from build123d import *

# Parameters (mm, degrees)
SKETCH1_W               = 120
SKETCH1_H               = 38
SKETCH1_W_2             = 41
SKETCH1_H_2             = 20
BOSS_EXTRUDE1_DEPTH     = 11
FILLET1_RADIUS          = 19
FILLET1_LENGTH          = 11
BOSS_EXTRUDE2_START     = 8
BOSS_EXTRUDE2_DEPTH     = 8
FILLET2_R               = 16
CUT_EXTRUDE2_DEPTH      = 66.741919656
CUT_EXTRUDE2_DEPTH_BACK = 66.741919656
BOSS_EXTRUDE3_START     = 8
BOSS_EXTRUDE3_OUTLINE_W = 32
BOSS_EXTRUDE3_OUTLINE_H = 8
BOSS_EXTRUDE3_DEPTH     = 49
SKETCH8_W               = 52
SKETCH8_H               = 38
BOSS_EXTRUDE4_DEPTH     = 8
SKETCH9_W               = 27
SKETCH9_H               = 38
CUT_EXTRUDE3_DEPTH      = 5
BOSS_EXTRUDE5_START     = -2
SKETCH11_W              = 41
SKETCH11_H              = 20
BOSS_EXTRUDE5_DEPTH     = 2
SKETCH13_R              = 6.5
CUT_EXTRUDE6_DEPTH      = 8
FILLET7_R               = 6
SKETCH25_R              = 2.15
CUT_EXTRUDE13_DEPTH     = 66.741919805
SKETCH10_W              = 38.2
SKETCH10_H              = 20
CUT_EXTRUDE14_DEPTH     = 74.518705262
BOSS_EXTRUDE6_DEPTH     = 1.5
LPATTERN1_COUNT         = 2
LPATTERN1_PITCH         = 39.5
SKETCH27_W              = 10
SKETCH27_H              = 8
BOSS_EXTRUDE7_DEPTH     = 27
FILLET8_R               = 3
CUT_EXTRUDE15_REACH     = 114.349
SKETCH28_R              = 2.15


# Read off the part's stored shape, not the designer's step: Boss-Extrude3
# Some blends are built 0.0001 mm under size
with BuildPart() as part:
    # Sketch1 → Boss-Extrude1 (new body)
    with BuildSketch(Plane.XY):
        Rectangle(SKETCH1_W, SKETCH1_H)
        with Locations((-24.5, 0)):
            Rectangle(SKETCH1_W_2, SKETCH1_H_2, mode=Mode.SUBTRACT)
    extrude(amount=BOSS_EXTRUDE1_DEPTH)

    # Fillet1: full round fillet: the end face becomes a half cylinder, R = half its width
    fillet1_face = Plane((-60, 0, 5.5), x_dir=(0, 0, 1), z_dir=(-1, 0, 0))  # on the end face: x along it, z out of the body
    fillet1_slab = fillet1_face.offset(-FILLET1_RADIUS / 2) * Box(FILLET1_LENGTH, 2 * FILLET1_RADIUS, FILLET1_RADIUS, mode=Mode.PRIVATE)  # the body's end, R deep
    fillet1_round = Plane((-41, 0, 5.5), x_dir=(-1, 0, 0), z_dir=(0, 0, 1)) * Cylinder(FILLET1_RADIUS, FILLET1_LENGTH, mode=Mode.PRIVATE)  # its axis R under the face
    add(fillet1_slab - fillet1_round, mode=Mode.SUBTRACT)

    # Sketch5 → Boss-Extrude2 (add)
    with BuildSketch(Plane.XY.offset(11).offset(BOSS_EXTRUDE2_START)):
        with BuildLine():
            Line((60, 19), (-41, 19))
            ThreePointArc((-41, 19), (-60, 0), (-41, -19))
            Line((-41, -19), (60, -19))
            Line((60, -19), (60, 19))
        make_face()
        with BuildLine():
            Line((57, 16), (-41, 16))
            ThreePointArc((-41, 16), (-57, 0), (-41, -16))
            Line((-41, -16), (57, -16))
            Line((57, -16), (57, 16))
        make_face(mode=Mode.SUBTRACT)
    extrude(amount=-BOSS_EXTRUDE2_DEPTH)

    # Fillet2
    fillet2_edges = [part.edges().sort_by_distance(p)[0] for p in [
        (57, 16, 15),
        (57, -16, 15),
    ]]
    fillet(fillet2_edges, radius=FILLET2_R - 0.0001)  # a hair under: the kernel refuses the full size

    # Sketch6 → Cut-Extrude2 (cut, two sides: drawn at the far end of the back side and taken through both)
    with BuildSketch(Plane(origin=(0, 0, 0), x_dir=(1, 0, 0), z_dir=(0, 1, 0)).offset(-CUT_EXTRUDE2_DEPTH_BACK)):
        with BuildLine():
            add(Edge.make_bspline(
                [(-60, -13.666666667), (-50.023022061, -12.774335398), (-44.35489615, -13.481329797), (-34.284055631, -17.771751053), (-23.960245459, -19), (-20, -19)],
                knots=[0, 0, 0, 0, 0.415410377, 0.639728072, 1, 1, 1, 1], degree=3))
            Line((-20, -19), (-60, -19))
            Line((-60, -19), (-60, -13.666666667))
        make_face()
    extrude(amount=CUT_EXTRUDE2_DEPTH + CUT_EXTRUDE2_DEPTH_BACK, mode=Mode.SUBTRACT)

    # Boss-Extrude3 outline → Boss-Extrude3 (add)
    with BuildSketch(Plane.YZ.offset(BOSS_EXTRUDE3_START)):
        with Locations((0, 15)):
            Rectangle(BOSS_EXTRUDE3_OUTLINE_W, BOSS_EXTRUDE3_OUTLINE_H)
    extrude(amount=BOSS_EXTRUDE3_DEPTH)

    # Sketch8 → Boss-Extrude4 (add)
    with BuildSketch(Plane(origin=(0, 0, 0), x_dir=(-1, 0, 0), z_dir=(0, 0, -1))):
        with Locations((-34, 0)):
            Rectangle(SKETCH8_W, SKETCH8_H)
    extrude(amount=BOSS_EXTRUDE4_DEPTH)

    # Sketch9 → Cut-Extrude3 (cut)
    with BuildSketch(Plane(origin=(60, 0, 0), x_dir=(0, 0, -1), z_dir=(1, 0, 0))):
        with Locations((-5.5, 0)):
            Rectangle(SKETCH9_W, SKETCH9_H)
    extrude(amount=-CUT_EXTRUDE3_DEPTH, mode=Mode.SUBTRACT)

    # Sketch11 → Boss-Extrude5 (add)
    with BuildSketch(Plane(origin=(0, 0, 0), x_dir=(-1, 0, 0), z_dir=(0, 0, -1)).offset(BOSS_EXTRUDE5_START)):
        with BuildLine():
            Line((-8, 19), (-8, -19))
            Line((-8, -19), (41, -19))
            ThreePointArc((41, -19), (60, 0), (41, 19))
            Line((41, 19), (-8, 19))
        make_face()
        with Locations((24.5, 0)):
            Rectangle(SKETCH11_W, SKETCH11_H, mode=Mode.SUBTRACT)
    extrude(amount=BOSS_EXTRUDE5_DEPTH)

    # Sketch13 → Cut-Extrude6 (cut)
    with BuildSketch(Plane(origin=(55, 0, 0), x_dir=(0, 0, -1), z_dir=(1, 0, 0))):
        with Locations(Location((-5.5, 5.3, 0), (0, 0, 90))):
            Circle(SKETCH13_R)
    extrude(amount=-CUT_EXTRUDE6_DEPTH, mode=Mode.SUBTRACT)

    # Fillet7
    fillet7_edges = [part.edges().sort_by_distance(p)[0] for p in [
        (8, 0, 0),
    ]]
    fillet(fillet7_edges, radius=FILLET7_R)

    # Sketch25 → Cut-Extrude13 (cut, through all)
    with BuildSketch(Plane.XY.offset(11)):
        with Locations((-49.85, 5)):
            Circle(SKETCH25_R)
        with Locations((-49.85, -5)):
            Circle(SKETCH25_R)
        with Locations((0.05, -5)):
            Circle(SKETCH25_R)
        with Locations((0.05, 5)):
            Circle(SKETCH25_R)
    extrude(amount=-CUT_EXTRUDE13_DEPTH, mode=Mode.SUBTRACT)

    # Sketch10 → Cut-Extrude14 (cut, through all)
    with BuildSketch(Plane.XZ.offset(19)):
        with Locations((35.9, 5.5)):
            Rectangle(SKETCH10_W, SKETCH10_H)
    extrude(amount=-CUT_EXTRUDE14_DEPTH, mode=Mode.SUBTRACT)

    # Sketch26 → Boss-Extrude6 (add)
    with BuildSketch(Plane.XZ.offset(19)):
        Polygon((8, -8), (55, -8), (55, -4.5), (16.8, -4.5), (16.8, 15.5), (55, 15.5), (55, 19), (8, 19), (8, -6), align=None)
    boss_extrude6 = extrude(amount=BOSS_EXTRUDE6_DEPTH)

    # LPattern1: Boss-Extrude6 ×2
    with Locations(*[(0, i * LPATTERN1_PITCH, 0) for i in range(1, LPATTERN1_COUNT)]):
        add(boss_extrude6)

    # Sketch27 → Boss-Extrude7 (add, through all)
    with BuildSketch(Plane.XY.offset(19)):
        with Locations((42, 24.5)):
            Rectangle(SKETCH27_W, SKETCH27_H)
        with Locations((42, -24.5)):
            Rectangle(SKETCH27_W, SKETCH27_H)
    extrude(amount=-BOSS_EXTRUDE7_DEPTH)

    # Fillet8
    # the kernel refuses this fillet: 3 mm, written as the material it takes off along each edge
    with BuildSketch(Plane(origin=(55, -28, 19), x_dir=(-1, 0, 0), z_dir=(0, 1, 0)), Plane(origin=(55, 28, -8), x_dir=(-1, 0, 0), z_dir=(0, -1, 0)), Plane(origin=(55, -28, 15.5), x_dir=(0, 0, 1), z_dir=(0, 1, 0))) as fillet8_piece_1:
        with BuildLine():
            CenterArc((FILLET8_R, -FILLET8_R), FILLET8_R, 90, 90)
            Line((0, -FILLET8_R), (0, 0))
            Line((0, 0), (FILLET8_R, 0))
        make_face()
    extrude(amount=56, mode=Mode.SUBTRACT)
    with BuildSketch(Plane(origin=(55, 28, -4.5), x_dir=(-1, 0, 0), z_dir=(0, -1, 0))) as fillet8_piece_2:
        with BuildLine():
            CenterArc((FILLET8_R, FILLET8_R), FILLET8_R, 180, 90)
            Line((0, FILLET8_R), (0, 0))
            Line((0, 0), (FILLET8_R, 0))
        make_face()
    extrude(amount=56, mode=Mode.SUBTRACT)
    with BuildSketch(Plane(origin=(47, 36, -8), x_dir=(-1, 0, 0), z_dir=(0, -1, 0)), Plane(origin=(47, -36, 19), x_dir=(-1, 0, 0), z_dir=(0, 1, 0))) as fillet8_piece_3:
        with BuildLine():
            CenterArc((FILLET8_R, -FILLET8_R), FILLET8_R, 90, 90)
            Line((0, -FILLET8_R), (0, 0))
            Line((0, 0), (FILLET8_R, 0))
        make_face()
    extrude(amount=15.5, mode=Mode.SUBTRACT)
    with BuildSketch(Plane(origin=(29.5, 28.5, -8), x_dir=(0, -1, 0), z_dir=(1, 0, 0)), Plane(origin=(29.5, -28.5, 19), x_dir=(0, 1, 0), z_dir=(1, 0, 0))) as fillet8_piece_4:
        with BuildLine():
            CenterArc((FILLET8_R, -FILLET8_R), FILLET8_R, 90, 90)
            Line((0, -FILLET8_R), (0, 0))
            Line((0, 0), (FILLET8_R, 0))
        make_face()
    extrude(amount=25, mode=Mode.SUBTRACT)
    with BuildSketch(Plane(origin=(47, 36, 19), x_dir=(-1, 0, 0), z_dir=(0, -1, 0)), Plane(origin=(47, -36, -8), x_dir=(-1, 0, 0), z_dir=(0, 1, 0))) as fillet8_piece_5:
        with BuildLine():
            CenterArc((FILLET8_R, FILLET8_R), FILLET8_R, 180, 90)
            Line((0, FILLET8_R), (0, 0))
            Line((0, 0), (FILLET8_R, 0))
        make_face()
    extrude(amount=15.5, mode=Mode.SUBTRACT)
    with BuildSketch(Plane(origin=(29.5, 28.5, 19), x_dir=(0, -1, 0), z_dir=(1, 0, 0)), Plane(origin=(29.5, -28.5, -8), x_dir=(0, 1, 0), z_dir=(1, 0, 0))) as fillet8_piece_6:
        with BuildLine():
            CenterArc((FILLET8_R, FILLET8_R), FILLET8_R, 180, 90)
            Line((0, FILLET8_R), (0, 0))
            Line((0, 0), (FILLET8_R, 0))
        make_face()
    extrude(amount=25, mode=Mode.SUBTRACT)

    # Sketch28 → Cut-Extrude15 (cut, up to next)
    with BuildSketch(Plane(origin=(47, 0, 0), x_dir=(0, 0, -1), z_dir=(1, 0, 0)), mode=Mode.PRIVATE) as cut_extrude15_sk1:
        with Locations((-10.5, 25.35)):
            Circle(SKETCH28_R)
    cut_extrude15_tool1 = extrude(cut_extrude15_sk1.sketch, amount=-CUT_EXTRUDE15_REACH, mode=Mode.PRIVATE) & part.part
    # Sketch28 → Cut-Extrude15 (cut, up to next)
    with BuildSketch(Plane(origin=(47, 0, 0), x_dir=(0, 0, -1), z_dir=(1, 0, 0)), mode=Mode.PRIVATE) as cut_extrude15_sk2:
        with Locations((-0.5, 25.35)):
            Circle(SKETCH28_R)
    cut_extrude15_tool2 = extrude(cut_extrude15_sk2.sketch, amount=-CUT_EXTRUDE15_REACH, mode=Mode.PRIVATE) & part.part
    # Sketch28 → Cut-Extrude15 (cut, up to next)
    with BuildSketch(Plane(origin=(47, 0, 0), x_dir=(0, 0, -1), z_dir=(1, 0, 0)), mode=Mode.PRIVATE) as cut_extrude15_sk3:
        with Locations((-0.5, -25.35)):
            Circle(SKETCH28_R)
    cut_extrude15_tool3 = extrude(cut_extrude15_sk3.sketch, amount=-CUT_EXTRUDE15_REACH, mode=Mode.PRIVATE) & part.part
    # Sketch28 → Cut-Extrude15 (cut, up to next)
    with BuildSketch(Plane(origin=(47, 0, 0), x_dir=(0, 0, -1), z_dir=(1, 0, 0)), mode=Mode.PRIVATE) as cut_extrude15_sk4:
        with Locations((-10.5, -25.35)):
            Circle(SKETCH28_R)
    cut_extrude15_tool4 = extrude(cut_extrude15_sk4.sketch, amount=-CUT_EXTRUDE15_REACH, mode=Mode.PRIVATE) & part.part
    add(cut_extrude15_tool1.solids().sort_by_distance((47, 25.35, 10.5))[0], mode=Mode.SUBTRACT)
    add(cut_extrude15_tool2.solids().sort_by_distance((47, 25.35, 0.5))[0], mode=Mode.SUBTRACT)
    add(cut_extrude15_tool3.solids().sort_by_distance((47, -25.35, 0.5))[0], mode=Mode.SUBTRACT)
    add(cut_extrude15_tool4.solids().sort_by_distance((47, -25.35, 10.5))[0], mode=Mode.SUBTRACT)


solid = part.part
Geometry: final body of the model. Coordinates: model frame, mm. A direction names the side the tool comes from. Coordinates: 2 decimals unless noted, no trailing zeros. Order: outer loops, then holes, each group sorted by start corner. A loop starts at its lowest first (then second) coordinate and runs counter-clockwise, first axis right, second up.
1) Set-up query: faces 4 (the cylindrical face through (46.14, 23.67, 18.1)), 5 (the cylindrical face through (53.64, -0.29, 15.99)), 6 (the flat face through (-45, 0, 5)), 7 (the cylindrical face through (46.14, -23.67, -7.1)). Return all of +Z, -Z, +X, -X, +Y, -Y with unobstructed straight access to the full face (end or side cutting, diameter ignored); none if empty.
Result sheet:
face 4: +Z, +X, +Y
face 5: +X, +Y, -Y
face 6: +Z, -Z
face 7: -Z, +X, -Y
2) Section C-C (x = 33.5). Return loops of the section in (y, z), then the cut area to 3 significant figures.
Result sheet:
outline: (-20.5, -8) - (20.5, -8) - (20.5, -4.5) - (-20.5, -4.5) - close; (-20.5, 15.5) - (20.5, 15.5) - (20.5, 19) - (-20.5, 19) - close
area: 287 mm2
3) Ray query, probe 1 along Y at (x, z) = (0.05, 7.25); probe 2 along Z at (x, y) = (27.5, -11); probe 3 along Y at (x, z) = (-49.85, 5). Return the intervals inside material, ascending.
Result sheet:
probe 1: y = -19 to -7.15, -2.85 to 2.85, 7.15 to 19
probe 2: z = -8 to -4.5, 15.5 to 19
probe 3: y = -16.81 to -7.15, -2.85 to 2.85, 7.15 to 16.81
4) Section A-A (z = 5). Return loops of the section in (x, y).
Result sheet:
outline: (-41, -19) - (8, -19) - (8, -20.5) - (16.8, -20.5) - (16.8, 20.5) - (8, 20.5) - (8, 19) - (-41, 19) arc R19 ccw to start; (37, -28.5) - (47, -28.5) - (47, -20.5) - (37, -20.5) - close; (37, 20.5) - (47, 20.5) - (47, 28.5) - (37, 28.5) - close; hole circle Ø4.3 at (-49.85, -5); hole circle Ø4.3 at (-49.85, 5); hole (-45, -10) - (-4, -10) - (-4, 10) - (-45, 10) - close; hole circle Ø4.3 at (0.05, -5); hole circle Ø4.3 at (0.05, 5)
5) Section B-B (x = 0.05). Return loops of the section in (y, z).
Result sheet:
outline: (-19, 0) - (-7.15, 0) - (-7.15, 11) - (-16, 11) - (-16, 19) - (-19, 19) - close; (-2.85, 0) - (2.85, 0) - (2.85, 11) - (-2.85, 11) - close; (7.15, 0) - (19, 0) - (19, 19) - (16, 19) - (16, 11) - (7.15, 11) - close
6) Draft query along Y for faces 1 (the cylindrical face through (53.6, 0.29, -7.54)), 2 (the flat face through (16, 20.5, 6)), 3 (the flat face through (35, 0, -4.5)). Return one class per face: released by +Y, released by -Y, zero draft, split by the parting line, or undercut.
Result sheet:
face 1: zero draft
face 2: released by +Y
face 3: undercut
7) First-contact query: P1, Ø6, axis at x = -14.5, y = 16.5, coming from the -Z side; P2, Ø3.5, axis at x = 0.05, y = 5, coming from the +Z side; P3, Ø1, axis at x = 12, z = 1, coming from the -Y side; P4, Ø7, axis at x = 0.05, y = -5, coming from the -Z side. Flat tips, straight axial feed; report the tip coordinate or a pass-through.
Result sheet:
P1: stops at z = 0
P2: passes through
P3: stops at y = -20.5
P4: stops at z = -0.2
8) Section D-D (x = -49.85). Give the number of separate pieces and of enclosed holes in the cut face, then the cut area to 3 significant figures.
Result sheet:
separate pieces: 3
enclosed holes: 0
area: 291 mm2
